```python
from build123d import *

# Parameters (mm, degrees)
SKETCH2_W             = 150
SKETCH2_H             = 100
BOSS_EXTRUDE1_DEPTH   = 50
CHAMFER1_SIZE         = 30
CHAMFER1_SIZE2        = 10
CHAMFER1_PART_2_SIZE  = 30
CHAMFER1_PART_2_SIZE2 = 10
CHAMFER1_PART_3_SIZE  = 30
CHAMFER1_PART_3_SIZE2 = 10
CHAMFER1_PART_4_SIZE  = 30
CHAMFER1_PART_4_SIZE2 = 10
CUT_EXTRUDE1_DEPTH    = 282
BOSS_EXTRUDE2_DEPTH   = 3
CUT_EXTRUDE2_DEPTH    = 1
SKETCH9_R             = 5
BOSS_EXTRUDE3_DEPTH   = 10


with BuildPart() as part:
    # Sketch2 → Boss-Extrude1 (new body)
    with BuildSketch(Plane.XY):
        Rectangle(SKETCH2_W, SKETCH2_H)
    extrude(amount=-BOSS_EXTRUDE1_DEPTH)

    # Chamfer1
    chamfer1_edges = [part.edges().sort_by_distance(p)[0] for p in [
        (0, -50, 0),
    ]]
    chamfer1_side = [part.faces().sort_by_distance(p)[0] for p in [
        (0, -50, -25),
    ]]
    chamfer(chamfer1_edges, length=CHAMFER1_SIZE, length2=CHAMFER1_SIZE2, reference=chamfer1_side[0])

    # Chamfer1 part 2
    chamfer1_part_2_edges = [part.edges().sort_by_distance(p)[0] for p in [
        (-75, 0, 0),
    ]]
    chamfer1_part_2_side = [part.faces().sort_by_distance(p)[0] for p in [
        (-75, 0, -25),
    ]]
    chamfer(chamfer1_part_2_edges, length=CHAMFER1_PART_2_SIZE, length2=CHAMFER1_PART_2_SIZE2, reference=chamfer1_part_2_side[0])

    # Chamfer1 part 3
    chamfer1_part_3_edges = [part.edges().sort_by_distance(p)[0] for p in [
        (0, 50, 0),
    ]]
    chamfer1_part_3_side = [part.faces().sort_by_distance(p)[0] for p in [
        (0, 50, -25),
    ]]
    chamfer(chamfer1_part_3_edges, length=CHAMFER1_PART_3_SIZE, length2=CHAMFER1_PART_3_SIZE2, reference=chamfer1_part_3_side[0])

    # Chamfer1 part 4
    chamfer1_part_4_edges = [part.edges().sort_by_distance(p)[0] for p in [
        (75, 0, 0),
    ]]
    chamfer1_part_4_side = [part.faces().sort_by_distance(p)[0] for p in [
        (75, 0, -25),
    ]]
    chamfer(chamfer1_part_4_edges, length=CHAMFER1_PART_4_SIZE, length2=CHAMFER1_PART_4_SIZE2, reference=chamfer1_part_4_side[0])

    # Sketch5 → Cut-Extrude1 (cut)
    with BuildSketch(Plane(origin=(75, 0, 0), x_dir=(0, 0, -1), z_dir=(1, 0, 0))):
        Polygon((30, -50), (30, 50), (81.32895228, 62.665959411), (65.838490403, -81.97874305), align=None)
    extrude(amount=-CUT_EXTRUDE1_DEPTH, mode=Mode.SUBTRACT)

    # Sketch6 → Boss-Extrude2 (add)
    with BuildSketch(Plane.XY):
        Polygon((-43.903010181, -25.827914317), (-46.403010181, -21.497787298), (-51.403010181, -21.497787298), (-53.903010181, -25.827914317), (-51.403010181, -30.158041336), (-46.403010181, -30.158041336), align=None)
        Polygon((43.903010181, 25.827914317), (46.403010181, 21.497787298), (51.403010181, 21.497787298), (53.903010181, 25.827914317), (51.403010181, 30.158041336), (46.403010181, 30.158041336), align=None)
        Polygon((46.403010181, -30.158041336), (43.903010181, -25.827914317), (46.403010181, -21.497787298), (51.403010181, -21.497787298), (53.903010181, -25.827914317), (51.403010181, -30.158041336), align=None)
        Polygon((-46.403010181, 21.497787298), (-51.403010181, 21.497787298), (-53.903010181, 25.827914317), (-51.403010181, 30.158041336), (-46.403010181, 30.158041336), (-43.903010181, 25.827914317), align=None)
    extrude(amount=BOSS_EXTRUDE2_DEPTH)

    # Sketch7 → Cut-Extrude2 (cut)
    with BuildSketch(Plane.XY.offset(3)):
        Polygon((-49.074995517, -20.874091647), (-48.315685666, -20.874091647), (-48.315685666, -25.776876491), (-43.576392296, -25.776876491), (-43.576392296, -26.601644718), (-48.315685666, -26.601644718), (-48.315685666, -31.504429563), (-49.074995517, -31.504429563), (-49.074995517, -26.601644718), (-53.814288887, -26.601644718), (-53.814288887, -25.776876491), (-49.074995517, -25.776876491), align=None)
        Polygon((48.315685666, -26.601644718), (48.315685666, -31.504429563), (49.074995517, -31.504429563), (49.074995517, -26.601644718), (53.814288887, -26.601644718), (53.814288887, -25.776876491), (49.074995517, -25.776876491), (49.074995517, -20.874091647), (48.315685666, -20.874091647), (48.315685666, -25.776876491), (43.576392296, -25.776876491), (43.576392296, -26.601644718), align=None)
        Polygon((-48.315685666, 26.601644718), (-48.315685666, 31.504429563), (-49.074995517, 31.504429563), (-49.074995517, 26.601644718), (-53.814288887, 26.601644718), (-53.814288887, 25.776876491), (-49.074995517, 25.776876491), (-49.074995517, 20.874091647), (-48.315685666, 20.874091647), (-48.315685666, 25.776876491), (-43.576392296, 25.776876491), (-43.576392296, 26.601644718), align=None)
        Polygon((49.074995517, 20.874091647), (48.315685666, 20.874091647), (48.315685666, 25.776876491), (43.576392296, 25.776876491), (43.576392296, 26.601644718), (48.315685666, 26.601644718), (48.315685666, 31.504429563), (49.074995517, 31.504429563), (49.074995517, 26.601644718), (53.814288887, 26.601644718), (53.814288887, 25.776876491), (49.074995517, 25.776876491), align=None)
    extrude(amount=-CUT_EXTRUDE2_DEPTH, mode=Mode.SUBTRACT)

    # Sketch9 → Boss-Extrude3 (add)
    with BuildSketch(Plane.XY):
        Circle(SKETCH9_R)
    extrude(amount=BOSS_EXTRUDE3_DEPTH)


solid = part.part
```
Here's how the part is built. I have some questions about the finished solid (model axes, mm). A direction names the side the tool comes from. Round coordinates to 2 decimals unless told otherwise and drop trailing zeros. Order: outer loops, then holes, each group sorted by start corner. A loop starts at its lowest first (then second) coordinate and runs counter-clockwise, first axis right, second up. Notation, with made-up numbers: (-17, 10.25) -> (12, 10.25) arc R21 ccw to (12, 15.25) -> close; hole circle Ø3 at (41, -3.75). An arc over 180 degrees is marked (long way). Use a Markdown table: item, result. Add a question column.
(1) For faces 1 (the face through (52.67, 27.96, 1.48)), 2 (the face through (-45.17, -28.02, 1.48)), 3 (the face through (-49, -30.158, 1)), 4 (the face through (-45.17, 28.02, 1.48)), 5 (the face through (-52.67, 27.96, 1.48)), which set-ups out of +Z, -Z, +X, -X, +Y, -Y let a thin tool reach every point of the face, with its end or its side?
(2) I need wall thicknesses on line 1 along Z through (x, y) = (43.5, 13.5); line 2 along Y through (x, z) = (-18.5, -7.5); line 3 along X through (y, z) = (-14, -6). Which ranges of each line are inside material? Lowest first, please.
(3) For pin 1 Ø2 at (x, z) = (49, -20.5) entering from +Y; pin 2 Ø3.5 at (x, y) = (52, -23.5) entering from +Z; pin 3 Ø5 at (x, z) = (27, -0.5) entering from -Y, each with a flat end and sliding along its axis, tell me the tip position at first contact or that it passes through.
(4) Suppose I cut it at C-C, the plane z = -10. Please give me the cut outline in (x, y), and give its area (3 significant figures).
(5) Suppose I cut it at B-B, the plane y = 0. Please give me the cut outline in (x, z), and give its area (3 significant figures).
(6) Suppose I cut it at D-D, the plane y = 23. Please give me the cut outline in (x, z) (3 decimals), and give its area (3 significant figures).
(7) If we mould it in two halves opening along Y, with no side actions, what happens to faces 6 (the face through (49, -26, 2)), 7 (the face through (49, 21.498, 1)), 8 (the face through (-1, -45, -15)), 9 (the face through (1, -1, -30))? For each: released by +Y, released by -Y, zero draft, split by the parting line, or undercut.
(8) Suppose I cut it at A-A, the plane x = 0. Please give me the cut outline in (y, z), and give its area (3 significant figures).
Verdict:
| question | item | result |
|---|---|---|
| 1 | face 1 | +Z, +X, +Y |
| 1 | face 2 | +Z, -Y |
| 1 | face 3 | +Z, +X, -X, -Y |
| 1 | face 4 | +Z, +Y |
| 1 | face 5 | +Z, -X, +Y |
| 2 | line 1 | -30 to 0 |
| 2 | line 2 | -42.5 to 42.5 |
| 2 | line 3 | -67 to 67 |
| 3 | pin 1 | y = 47.17 |
| 3 | pin 2 | z = 3 |
| 3 | pin 3 | y = -41 |
| 4 | outline | (-68.33, -43.33) -> (68.33, -43.33) -> (68.33, 43.33) -> (-68.33, 43.33) -> close |
| 4 | area | 11,800 mm2 |
| 5 | outline | (-75, -30) -> (75, -30) -> (65, 0) -> (5, 0) -> (5, 10) -> (-5, 10) -> (-5, 0) -> (-65, 0) -> close |
| 5 | area | 4,300 mm2 |
| 6 | outline | (-75, -30) -> (75, -30) -> (65, 0) -> (52.27, 0) -> (52.27, 3) -> (49.075, 3) -> (49.075, 2) -> (48.316, 2) -> (48.316, 3) -> (45.536, 3) -> (45.536, 0) -> (-45.536, 0) -> (-45.536, 3) -> (-48.316, 3) -> (-48.316, 2) -> (-49.075, 2) -> (-49.075, 3) -> (-52.27, 3) -> (-52.27, 0) -> (-65, 0) -> close |
| 6 | area | 4,240 mm2 |
| 7 | face 6 | undercut |
| 7 | face 7 | undercut |
| 7 | face 8 | released by -Y |
| 7 | face 9 | zero draft |
| 8 | outline | (-50, -30) -> (50, -30) -> (40, 0) -> (5, 0) -> (5, 10) -> (-5, 10) -> (-5, 0) -> (-40, 0) -> close |
| 8 | area | 2,800 mm2 |
